Input: part model. Units: mm. Frame: model coordinates. A direction names the side the tool comes from. Coordinates: 2 decimals unless noted, no trailing zeros. Loops run counter-clockwise (first coordinate to the right, second up) from the corner with the lowest first, then second, coordinate; pieces in that order, holes last.
```python
from build123d import *

# Parameters (mm, degrees)
SKETCH_1_W               = 73.73
SKETCH_1_H               = 66.24
EXTRUDE_1_DEPTH          = 11
CUT_EXTRUDE_1_DEPTH      = 14
CUT_EXTRUDE_1_DEPTH_BACK = 100.723871265
SKETCH_5_R               = 1.6
CUT_EXTRUDE_2_DEPTH      = 9.5
SKETCH_8_R               = 0.5
SKETCH_8_R_2             = 0.499999992
SKETCH_8_R_3             = 2.25
SKETCH_8_R_4             = 6
CUT_EXTRUDE_3_DEPTH      = 9
CUT_EXTRUDE_4_DEPTH      = 9
SKETCH_11_W              = 28.050882838
SKETCH_11_H              = 6.729999604
CUT_EXTRUDE_5_DEPTH      = 9
FILLET_1_R               = 5


with BuildPart() as part:
    # 草图1 → 凸台-拉伸1 (new body)
    with BuildSketch(Plane.XY):
        with Locations((36.865, 33.12)):
            Rectangle(SKETCH_1_W, SKETCH_1_H)
    extrude(amount=EXTRUDE_1_DEPTH)

    # 草图5 → 切除-拉伸1 (cut, two sides: drawn at the far end of the back side and taken through both)
    with BuildSketch(Plane.XY.offset(-CUT_EXTRUDE_1_DEPTH_BACK)):
        with Locations(Location((5.115, 61.125, 0), (0, 0, 180))):
            Circle(SKETCH_5_R)
        with Locations(Location((68.615, 61.125, 0), (0, 0, 180))):
            Circle(SKETCH_5_R)
        with Locations(Location((68.615, 5.115, 0), (0, 0, 180))):
            Circle(SKETCH_5_R)
        with Locations(Location((5.115, 5.115, 0), (0, 0, 180))):
            Circle(SKETCH_5_R)
    extrude(amount=CUT_EXTRUDE_1_DEPTH + CUT_EXTRUDE_1_DEPTH_BACK, mode=Mode.SUBTRACT)

    # 草图6 → 切除-拉伸2 (cut)
    with BuildSketch(Plane.XY.offset(11)):
        with BuildLine():
            Line((1.36, 58.125), (1.36, 8.115))
            Line((1.36, 8.115), (5.115, 8.115))
            ThreePointArc((5.115, 8.115), (7.236320344, 7.236320344), (8.115, 5.115))
            Line((8.115, 5.115), (8.115, 1.36))
            Line((8.115, 1.36), (65.615, 1.36))
            Line((65.615, 1.36), (65.615, 5.115))
            ThreePointArc((65.615, 5.115), (66.493679656, 7.236320344), (68.615, 8.115))
            Line((68.615, 8.115), (72.37, 8.115))
            Line((72.37, 8.115), (72.37, 58.125))
            Line((72.37, 58.125), (68.615, 58.125))
            ThreePointArc((68.615, 58.125), (66.493679656, 59.003679656), (65.615, 61.125))
            Line((65.615, 61.125), (65.615, 64.88))
            Line((65.615, 64.88), (8.115, 64.88))
            Line((8.115, 64.88), (8.115, 61.125))
            ThreePointArc((8.115, 61.125), (7.236320344, 59.003679656), (5.115, 58.125))
            Line((5.115, 58.125), (1.36, 58.125))
        make_face()
    extrude(amount=-CUT_EXTRUDE_2_DEPTH, mode=Mode.SUBTRACT)

    # 草图8 → 切除-拉伸3 (cut)
    with BuildSketch(Plane.XY):
        with Locations(Location((62.581524864, 61.690056586, 0), (0, 0, 180))):
            Circle(SKETCH_8_R)
        with Locations(Location((60.543023731, 61.690056586, 0), (0, 0, 180))):
            Circle(SKETCH_8_R_2)
        with Locations(Location((64.607021964, 61.690056586, 0), (0, 0, 180))):
            Circle(SKETCH_8_R)
        with Locations(Location((54.862855038, 58.701240743, 0), (0, 0, 180))):
            Circle(SKETCH_8_R_3)
        with Locations(Location((49.528855397, 58.701240743, 0), (0, 0, 180))):
            Circle(SKETCH_8_R_3)
        with Locations(Location((40.365063963, 61.690056586, 0), (0, 0, 180))):
            Circle(SKETCH_8_R)
        with Locations(Location((13.058538298, 21.432969982, 0), (0, 0, 180))):
            Circle(SKETCH_8_R_4)
    extrude(amount=CUT_EXTRUDE_3_DEPTH, mode=Mode.SUBTRACT)

    # 草图10 → 切除-拉伸4 (cut)
    with BuildSketch(Plane(origin=(0, 66.24, 0), x_dir=(1, 0, 0), z_dir=(0, 1, 0))):
        with BuildLine():
            Line((17.808167787, -6.98156116), (9.328167793, -6.98156116))
            ThreePointArc((9.328167793, -6.98156116), (8.621061012, -7.274454379), (8.328167793, -7.98156116))
            Line((8.328167793, -7.98156116), (8.328167793, -11))
            Line((8.328167793, -11), (18.808167787, -11))
            Line((18.808167787, -11), (18.808167787, -7.98156116))
            ThreePointArc((18.808167787, -7.98156116), (18.515274569, -7.274454379), (17.808167787, -6.98156116))
        make_face()
    extrude(amount=-CUT_EXTRUDE_4_DEPTH, mode=Mode.SUBTRACT)

    # 草图11 → 切除-拉伸5 (cut)
    with BuildSketch(Plane.XZ):
        with Locations((21.447326516, 7.836561358)):
            Rectangle(SKETCH_11_W, SKETCH_11_H)
    extrude(amount=-CUT_EXTRUDE_5_DEPTH, mode=Mode.SUBTRACT)

    # 圆角1
    fillet_1_edges = [part.edges().sort_by_distance(p)[0] for p in [
        (0, 66.24, 5.5),
        (73.73, 66.24, 5.5),
        (73.73, 0, 5.5),
        (0, 0, 5.5),
    ]]
    fillet(fillet_1_edges, radius=FILLET_1_R)


solid = part.part
```
Item 1: Mould query, pull axis X, two halves, no side actions, for faces 3 (the face through (72.2, 1.4, 5.6)), 4 (the face through (1, 33, 11)), 5 (the face through (5.32, 59.54, 5.42)). Classes: +X half, -X half, draft (parallel to the pull), parting line (faces both ways), or undercut.
Result:
face 3: +X half
face 4: draft
face 5: undercut
Item 2: Section query D-D (x = 37). Output: boundary loops of the cut face in (y, z), then the cut area to 3 significant figures.
Result:
outline: (0, 0) - (66.24, 0) - (66.24, 11) - (64.88, 11) - (64.88, 1.5) - (1.36, 1.5) - (1.36, 11) - (0, 11) - close
area: 125 mm2
Item 3: Section query B-B (y = 45). Output: boundary loops of the cut face in (x, z).
Result:
outline: (0, 0) - (73.73, 0) - (73.73, 11) - (72.37, 11) - (72.37, 1.5) - (1.36, 1.5) - (1.36, 11) - (0, 11) - close
Item 4: Section query C-C (x = 10.5). Output: boundary loops of the cut face in (y, z).
Result:
outline: (0, 0) - (16.01, 0) - (16.01, 1.5) - (1.36, 1.5) - (1.36, 4.47) - (0, 4.47) - close; (26.86, 0) - (66.24, 0) - (66.24, 6.98) - (64.88, 6.98) - (64.88, 1.5) - (26.86, 1.5) - close
Item 5: Reachability of faces 1 (the face through (4.25, 3.77, 5.42)), 2 (the face through (3, 8.115, 6)) from +Z, -Z, +X, -X, +Y, -Y: full face, straight path, thin tool, end or side. Return the list, or none.
Result:
face 1: +Z, -Z
face 2: +Z
Item 6: Section query A-A (z = 10). Count the separate pieces of the cut face and the enclosed holes in it, then the cut area to 3 significant figures.
Result:
separate pieces: 2
enclosed holes: 4
area: 439 mm2
Item 7: Contact query for flat-ended pins moving along their axis: P1, Ø4, axis at x = 49.53, y = 58.7, coming from the -Z side; P2, Ø1, axis at x = 64, y = 12, coming from the -Z side; P3, Ø1.1, axis at y = 62.5, z = 5.5, coming from the +X side; P4, Ø0.9, axis at y = 3.5, z = 3.5, coming from the +X side. Output: stop coordinate, or through.
Result:
P1: passes through
P2: stops at z = 0
P3: stops at x = 73.68
P4: stops at x = 73.62
Item 8: Line query: L1, parallel to X at y = 27, z = 7.5; L2, parallel to Y at x = 62.5, z = 1; L3, parallel to Y at x = 51.5, z = 1.75. Output: solid intervals per line, ascending.
Result:
L1: x = 0 to 1.36, 72.37 to 73.73
L2: y = 0 to 61.2, 62.18 to 66.24
L3: y = 0 to 1.36, 64.88 to 66.24
